from build123d import *

# Parameters (mm, degrees)
ESQUISSE1_R        = 1.5
BOSS_EXTRU_1_DEPTH = 3
ESQUISSE3_R        = 3
ESQUISSE3_R_2      = 1
BOSS_EXTRU_2_DEPTH = 10
CONG_1_R           = 5
BOSS_EXTRU_3_DEPTH = 3


with BuildPart() as part:
    # Esquisse1 → Boss.-Extru.1 (new body)
    with BuildSketch(Plane.XY):
        Polygon((0, 27), (0, 0), (5.65, 0), (7.65, 0), (7.700374591, 0), (16.027478889, 0), (33.35, 0), (35.35, 0), (41, 0), (41, 27), (30.5, 27), (30.5, 3.727272727), (10.5, 3.727272727), (10.5, 27), align=None)
        with Locations((4, 3.498076118)):
            Circle(ESQUISSE1_R, mode=Mode.SUBTRACT)
        with Locations((36.99999993, 3.500228257)):
            Circle(ESQUISSE1_R, mode=Mode.SUBTRACT)
        with Locations((4, 23.998076118)):
            Circle(ESQUISSE1_R, mode=Mode.SUBTRACT)
        with Locations((36.99999993, 23.998304375)):
            Circle(ESQUISSE1_R, mode=Mode.SUBTRACT)
    extrude(amount=BOSS_EXTRU_1_DEPTH)

    # Esquisse3 → Boss.-Extru.2 (add)
    with BuildSketch(Plane.XY.offset(3)):
        with Locations((6.5, 14)):
            Circle(ESQUISSE3_R)
        with Locations((6.5, 14)):
            Circle(ESQUISSE3_R_2, mode=Mode.SUBTRACT)
        with Locations((34.5, 14)):
            Circle(ESQUISSE3_R)
        with Locations((34.5, 14)):
            Circle(ESQUISSE3_R_2, mode=Mode.SUBTRACT)
    extrude(amount=BOSS_EXTRU_2_DEPTH)

    # Congé1
    cong_1_edges = [part.edges().sort_by_distance(p)[0] for p in [
        (30.5, 27, 1.5),
        (41, 27, 1.5),
        (41, 0, 1.5),
        (0, 0, 1.5),
        (0, 27, 1.5),
        (10.5, 27, 1.5),
    ]]
    fillet(cong_1_edges, radius=CONG_1_R)

    # Esquisse5 → Boss.-Extru.3 (add)
    with BuildSketch(Plane.XY.offset(3)):
        Polygon((8, 0), (6, 0), (6, -28.26), (35.7, -28.26), (35.7, 0), (33.7, 0), (33.7, -26.26), (8, -26.26), align=None)
    extrude(amount=-BOSS_EXTRU_3_DEPTH)


solid = part.part
Can you work these out from the model? Positions are in its coordinate system, mm. A direction names the side the tool comes from. Give positions to 0.01 mm unless a question says otherwise; leave off trailing zeros. Order: outer loops, then holes, each group sorted by start corner. A loop starts at its lowest first (then second) coordinate and runs counter-clockwise, first axis right, second up. Notation, with made-up numbers: M 89,80.25 L 134,80.25 A19 ccw 134,112.25 Z; hole C -27,-28 d9. An arc over 180 degrees is marked long. One line per item, written item: value.
Item 1: If we mould it in two halves opening along Y, with no side actions, what happens to faces 5 (the face through (6, 14, 3)), 6 (the face through (35.7, -14, 2)), 7 (the face through (7.884, 11.338, 7.93))? For each: pulls with the +Y half, pulls with the -Y half, needs draft (parallel to the pull), parting line crosses it, or undercut.
Verdict:
face 5: undercut
face 6: needs draft
face 7: parting line crosses it
Item 2: If we section it at D-D on x = 34.5: Write out the boundary of the cut face in (y, z).
Verdict:
outline: M -28.26,0 L 26.9,0 L 26.9,3 L 17,3 L 17,13 L 15,13 L 15,3 L 13,3 L 13,13 L 11,13 L 11,3 L -28.26,3 Z
Item 3: If we section it at A-A on y = 14: Write out the boundary of the cut face in (x, z).
Verdict:
outline: M 0,0 L 10.5,0 L 10.5,3 L 9.5,3 L 9.5,13 L 7.5,13 L 7.5,3 L 5.5,3 L 5.5,13 L 3.5,13 L 3.5,3 L 0,3 Z; M 30.5,0 L 41,0 L 41,3 L 37.5,3 L 37.5,13 L 35.5,13 L 35.5,3 L 33.5,3 L 33.5,13 L 31.5,13 L 31.5,3 L 30.5,3 Z
Item 4: If we section it at C-C on z = 9.75: Write out the boundary of the cut face in (x, y), and give its area (3 significant figures).
Verdict:
outline: C 6.5,14 d6; C 34.5,14 d6; hole C 6.5,14 d2; hole C 34.5,14 d2
area: 50.3 mm2
Item 5: For pin 1 (2 mm diameter, centred on x = 4.5, z = 11.5, fed in from -Y); pin 2 (2.5 mm diameter, centred on y = -17.5, z = 2, fed in from -X); pin 3 (10 mm diameter, centred on x = 30.5, y = -5, fed in from +Z), each with a flat end and sliding along its axis, tell me the tip position at first contact or that it passes through.
Verdict:
pin 1: y = 11.17
pin 2: x = 6
pin 3: z = 3
Item 6: For faces 1 (the face through (32, 25.57, 1.52)), 2 (the face through (21, 0, 1)), 3 (the face through (21, -28.26, 2)), 4 (the face through (34.96, 13.11, 7.93)), which set-ups out of +Z, -Z, +X, -X, +Y, -Y let a thin tool reach every point of the face, with its end or its side?
Verdict:
face 1: +Z, -Z, +Y
face 2: +Z, -Z
face 3: +Z, -Z, +X, -X, -Y
face 4: +Z
Item 7: Please list where these lines run through material, in increasing order: line 1 (Y direction, x = 4, z = 1.4); line 2 (X direction, y = 11, z = 1.75); line 3 (Z direction, x = 3, y = 13.5).
Verdict:
line 1: 0.1 to 2, 5 to 22.5, 25.5 to 26.9
line 2: 0 to 10.5, 30.5 to 41
line 3: 0 to 3
Item 8: If we section it at B-B on x = 19: Write out the boundary of the cut face in (y, z), and give its area (3 significant figures).
Verdict:
outline: M -28.26,0 L -26.26,0 L -26.26,3 L -28.26,3 Z; M 0,0 L 3.73,0 L 3.73,3 L 0,3 Z
area: 17.2 mm2
